Could you check a few things on this model? Use its own coordinates, in mm. A direction names the side the tool comes from. Give positions to 0.01 mm unless a question says otherwise; leave off trailing zeros. Write each loop counter-clockwise with the first axis right and the second up, starting at its lowest first coordinate (ties: lowest second). Pieces come first, ordered by that corner, then holes. Notation, with made-up numbers: (-28, -0.5) - (-11, -0.5) arc R21 cw to (-11, 33.5) - close; hole circle Ø1 at (81.5, 43). An arc over 180 degrees is marked (long way). Answer as a JSON object with one key per item and string values. Group by question number.
Autodesk Inventor part; units mm, degrees
ref_plane "YZ Plane" through (0, 0, 0) normal (1, 0, 0) x (0, 1, 0)
ref_plane "XZ Plane" through (0, 0, 0) normal (0, 1, 0) x (-1, 0, 0)
ref_plane "XY Plane" through (0, 0, 0) normal (0, 0, 1) x (1, 0, 0)
sketch "Sketch1" plane through (0, 0, 0) normal (0, 1, 0) x (-1, 0, 0)
  line L0 (133.35, 82.55) -> (-133.35, 82.55)
  line L1 (-133.35, 82.55) -> (-133.35, -82.55)
  line L2 (-133.35, -82.55) -> (133.35, -82.55)
  line L3 (133.35, -82.55) -> (133.35, 82.55)
  line L4 (133.35, 82.55) -> (-133.35, -82.55) construction
  line L5 (-133.35, 82.55) -> (133.35, -82.55) construction
  line L6 (-150.8125, 104.775) -> (150.8125, 104.775)
  line L7 (150.8125, 104.775) -> (150.8125, -104.775)
  line L8 (150.8125, -104.775) -> (-150.8125, -104.775)
  line L9 (-150.8125, -104.775) -> (-150.8125, 104.775)
  line L10 (-150.8125, 104.775) -> (150.8125, -104.775) construction
  line L11 (150.8125, 104.775) -> (-150.8125, -104.775) construction
  point P0 (0, 0)
  dimension "d0" = 165.1
  dimension "d1" = 266.7
  dimension "d2" = 209.55
  dimension "d3" = 301.625
extrude "Extrusion1" add sketch "Sketch1" along normal blind 146.05
sketch "Sketch2" plane through (0, 0, 0) normal (0, -1, 0) x (1, 0, 0)
  line L0 (133.35, 82.55) -> (-133.35, 82.55)
  line L1 (-133.35, -82.55) -> (133.35, -82.55)
  line L2 (-133.35, 82.55) -> (133.35, 82.55)
  line L3 (133.35, 82.55) -> (133.35, -82.55)
  line L4 (133.35, -82.55) -> (-133.35, -82.55)
  line L5 (-133.35, -82.55) -> (-133.35, 82.55)
  point P0 (0, 0)
  point P1 (133.35, 82.55)
  point P2 (-133.35, -82.55)
extrude "Extrusion2" add sketch "Sketch2" against normal blind 3.175
sketch "Sketch3" plane through (0, 3.175, 0) normal (0, 1, 0) x (1, 0, 0)
  line L0 (-133.35, -82.55) -> (-133.35, 82.55)
  line L1 (-133.35, 82.55) -> (133.35, 82.55)
  line L2 (-133.35, -82.55) -> (133.35, -82.55)
  line L3 (133.35, -82.55) -> (133.35, 82.55)
  line L4 (133.35, 82.55) -> (-133.35, 82.55)
  line L5 (-133.35, 82.55) -> (-133.35, -82.55)
  line L6 (130.175, -79.375) -> (-130.175, -79.375)
  line L7 (-130.175, -79.375) -> (-130.175, 79.375)
  line L8 (-130.175, 79.375) -> (130.175, 79.375)
  line L9 (130.175, 79.375) -> (130.175, -79.375)
  point P0 (0, 0)
  dimension "d8" = 3.175
extrude "Extrusion3" add sketch "Sketch3" along normal blind 6.35 contours L6 L7 L8 L9
sketch "Sketch5" plane through (-133.35, 146.05, 82.55) normal (1, 0, 0) x (0, 0, -1)
  line L0 (0, -38.481) -> (165.1, -38.481)
  line L1 (165.1, -38.481) -> (14.224, -38.481)
  line L2 (14.224, -38.481) -> (14.224, -136.525)
  line L3 (14.224, -136.525) -> (165.1, -136.525)
  line L4 (165.1, -136.525) -> (165.1, -38.481)
  point P0 (82.55, -146.05)
  point P1 (165.1, -142.875)
  dimension "d15" = 98.044
  dimension "d16" = 150.876
  dimension "d19" = 6.35
extrude "Extrusion5" add sketch "Sketch5" along normal blind 92.964
sketch "Sketch6" plane through (0, 9.525, 0) normal (0, 1, 0) x (1, 0, 0)
  line L0 (62.8142, 28.702) -> (-34.036, 28.702)
  line L1 (-34.036, 28.702) -> (-34.036, -79.375)
  line L2 (-34.036, -79.375) -> (62.8142, -79.375)
  line L3 (62.8142, -79.375) -> (62.8142, 28.702)
  line L4 (-130.175, -79.375) -> (130.175, -79.375)
  line L5 (-40.386, 82.55) -> (-40.386, -68.326)
  point P0 (0, 0)
  dimension "d20" = 108.077
  dimension "d21" = 96.8502
  dimension "d61" = 0
  dimension "d62" = 6.35
extrude "Extrusion6" add sketch "Sketch6" along normal blind 3.175
sketch "Sketch8" plane through (0, 0, 0) normal (0, -1, 0) x (1, 0, 0)
  circle A0 centre (144.4625, 38.1) radius 3.4925
  line L0 (-150.8125, 104.775) -> (150.8125, 104.775)
  line L1 (150.8125, 104.775) -> (150.8125, -104.775)
  circle A1 centre (144.4625, -38.1) radius 3.4925
  line L2 (150.8125, -104.775) -> (-150.8125, -104.775)
  circle A2 centre (-144.4625, 38.1) radius 3.175
  circle A3 centre (-144.4625, -38.1) radius 3.4925
  line L3 (-150.8125, -104.775) -> (-150.8125, 104.775)
  line L4 (150.8125, 50.8) -> (-150.8125, 50.8)
  line L5 (150.8125, -50.8) -> (-150.8125, -50.8)
  point P0 (0, 0)
  dimension "d28" = 6.985
  dimension "d30" = 6.35
  dimension "d31" = 6.35
  dimension "d33" = 6.985
  dimension "d34" = 6.35
  dimension "d36" = 6.35
  dimension "d38" = 6.985
  dimension "d39" = 6.35
  dimension "d55" = 50.8
  dimension "d56" = 50.8
  dimension "d57" = 12.7
  dimension "d58" = 12.7
  dimension "d59" = 12.7
  dimension "d60" = 12.7
extrude "Extrusion8" cut sketch "Sketch8" against normal blind 6.35 contours A0 | A1 | A2 | A3
sketch "Sketch11" plane through (0, 12.7, 0) normal (0, 1, 0) x (1, 0, 0)
  circle A0 centre (56.2991, 19.7485) radius 1.7018
  circle A1 centre (56.2991, -70.4215) radius 1.7018
  circle A2 centre (-27.5209, 19.7485) radius 1.7018
  circle A3 centre (-27.5209, -70.4215) radius 1.7018
  line L0 (62.8142, 28.702) -> (-34.036, 28.702)
  line L1 (-34.036, -79.375) -> (62.8142, -79.375)
  line L2 (62.8142, -79.375) -> (62.8142, 28.702)
  line L3 (-34.036, 28.702) -> (-34.036, -79.375)
  point P0 (0, 0)
  dimension "d82" = 3.4036
  dimension "d83" = 83.82
  dimension "d85" = 83.82
  dimension "d87" = 6.5151
  dimension "d88" = 6.5151
  dimension "d89" = 90.17
  dimension "d90" = 8.9535
  dimension "d91" = 3.4036
  dimension "d92" = 3.4036
  dimension "d93" = 3.4036
extrude "Extrusion11" cut sketch "Sketch11" against normal up to surface (3.175 mm away) contours A0 | A1 | A2 | A3
sketch "Sketch12" plane through (-150.8125, 0, 104.775) normal (0, 0, 1) x (1, 0, 0)
  circle A0 centre (200.025, 89.154) radius 6.35
  line L0 (301.625, 0) -> (301.625, 146.05)
  line L1 (0, 146.05) -> (301.625, 146.05)
  point P0 (150.8125, 0)
  dimension "d77" = 12.7
  dimension "d78" = 101.6
  dimension "d79" = 56.896
extrude "Extrusion12" cut sketch "Sketch12" against normal up to surface (22.225 mm away)
properties part number "JunctionBox" material "ABS Plastic"
(1) Will these pins go through, and if not, where does the flat tip stop? P1, Ø7.5, axis at x = 49.21, y = 89.15, coming from the +Z side; P2, Ø8, axis at x = -5.5, z = -6.5, coming from the -Y side; P3, Ø1.7, axis at x = 56, z = 71, coming from the +Y side (3 decimals); P4, Ø4.5, axis at x = 56.3, z = 70.42, coming from the +Y side.
(2) For faces 5 (the flat face through (56, 9.525, -36)), 6 (the cylindrical face through (144.008, 3.131, 41.563)), 7 (the flat face through (-132, 9.525, -40)), which set-ups out of +Z, -Z, +X, -X, +Y, -Y let a thin tool reach every point of the face, with its end or its side?
(3) I need wall thicknesses on L1, parallel to X at y = 1, z = 38; L2, parallel to Z at x = -88.5, y = 6.5 (3 decimals); L3, parallel to Z at x = 122, y = 105.5 (3 decimals). Which ranges of each line are inside material? Lowest first, please.
(4) If we mould it in two halves opening along Z, with no side actions, what happens to faces 1 (the flat face through (23, 146.05, -85)), 2 (the flat face through (-2, 72, -104.775)), 3 (the flat face through (2, 72, 104.775)), 4 (the flat face through (130.175, 6, -1))? For each: +Z half, -Z half, draft (parallel to the pull), parting line (faces both ways), or undercut.
(5) I want a section at C-C, the plane x = 12. Please give me the cut outline in (y, z) (3 decimals).
(6) I want a section at D-D, the plane x = -54. Please give me the cut outline in (y, z) (3 decimals).
Entries:
{
 "1": {"P1": "z = -82.55", "P2": "y = 0", "P3": "y = 9.525", "P4": "y = 12.7"},
 "2": {"face 5": "+Y", "face 6": "-Y", "face 7": "none"},
 "3": {"L1": "-150.81 to -147.64, -141.29 to 140.97, 147.95 to 150.81", "L2": "-104.775 to -82.55, -79.375 to 79.375, 82.55 to 104.775", "L3": "-104.775 to -82.55, 82.55 to 104.775"},
 "4": {"face 1": "draft", "face 2": "-Z half", "face 3": "+Z half", "face 4": "undercut"},
 "5": {"outline": "(0, -104.775) - (146.05, -104.775) - (146.05, -82.55) - (3.175, -82.55) - (3.175, -79.375) - (9.525, -79.375) - (9.525, -28.702) - (12.7, -28.702) - (12.7, 79.375) - (3.175, 79.375) - (3.175, 82.55) - (146.05, 82.55) - (146.05, 104.775) - (0, 104.775) - close"},
 "6": {"outline": "(0, -104.775) - (146.05, -104.775) - (146.05, -82.55) - (107.569, -82.55) - (107.569, 68.326) - (9.525, 68.326) - (9.525, 79.375) - (3.175, 79.375) - (3.175, 82.55) - (146.05, 82.55) - (146.05, 104.775) - (0, 104.775) - close; hole (3.175, -82.55) - (9.525, -82.55) - (9.525, -79.375) - (3.175, -79.375) - close"}
}
